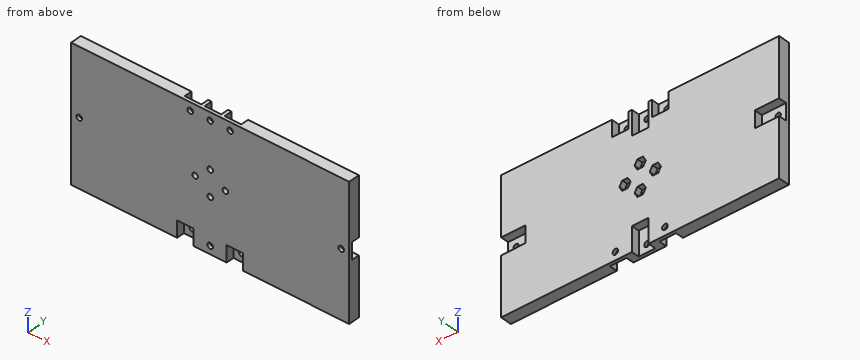
from build123d import *

# Parameters (mm, degrees)
SKETCH1_W           = 174.17
SKETCH1_H           = 83
BOSS_EXTRUDE1_DEPTH = 7
SKETCH2_R           = 1.75
CUT_EXTRUDE1_DEPTH  = 8
SKETCH3_R           = 1.75
CUT_EXTRUDE2_DEPTH  = 8
SKETCH4_W           = 15.4
SKETCH4_H           = 10.4
SKETCH4_W_2         = 10.4
SKETCH4_H_2         = 15.4
CUT_EXTRUDE3_DEPTH  = 5
SKETCH5_W           = 10.4
SKETCH5_H           = 10.4
CUT_EXTRUDE4_DEPTH  = 5
SKETCH6_R           = 1.75
CUT_EXTRUDE5_DEPTH  = 3
CUT_EXTRUDE6_DEPTH  = 3.64
SKETCH9_W           = 10.4
SKETCH9_H           = 10.4
CUT_EXTRUDE7_DEPTH  = 5
SKETCH10_R          = 1.75
CUT_EXTRUDE8_DEPTH  = 3


with BuildPart() as part:
    # Sketch1 → Boss-Extrude1 (new body)
    with BuildSketch(Plane(origin=(0, 0, 0), x_dir=(1, 0, 0), z_dir=(0, 1, 0))):
        with Locations((87.085, 41.5)):
            Rectangle(SKETCH1_W, SKETCH1_H)
    extrude(amount=BOSS_EXTRUDE1_DEPTH)

    # Sketch2 → Cut-Extrude1 (cut, through all)
    with BuildSketch(Plane(origin=(0, 7, 0), x_dir=(1, 0, 0), z_dir=(0, 1, 0))):
        with Locations((87.085, 49.5)):
            Circle(SKETCH2_R)
        with Locations((77.585, 41.5)):
            Circle(SKETCH2_R)
        with Locations((96.585, 41.5)):
            Circle(SKETCH2_R)
        with Locations((87.085, 33.5)):
            Circle(SKETCH2_R)
    extrude(amount=-CUT_EXTRUDE1_DEPTH, mode=Mode.SUBTRACT)

    # Sketch3 → Cut-Extrude2 (cut, through all)
    with BuildSketch(Plane(origin=(0, 7, 0), x_dir=(1, 0, 0), z_dir=(0, 1, 0))):
        with Locations((87.085, 78)):
            Circle(SKETCH3_R)
        with Locations((5, 41.5)):
            Circle(SKETCH3_R)
        with Locations((87.085, 5)):
            Circle(SKETCH3_R)
        with Locations((169.17, 41.5)):
            Circle(SKETCH3_R)
    extrude(amount=-CUT_EXTRUDE2_DEPTH, mode=Mode.SUBTRACT)

    # Sketch4 → Cut-Extrude3 (cut)
    with BuildSketch(Plane(origin=(0, 7, 0), x_dir=(1, 0, 0), z_dir=(0, 1, 0))):
        with Locations((7.5, 41.5)):
            Rectangle(SKETCH4_W, SKETCH4_H)
        with Locations((87.085, 7.5)):
            Rectangle(SKETCH4_W_2, SKETCH4_H_2)
        with Locations((87.085, 75.5)):
            Rectangle(SKETCH4_W_2, SKETCH4_H_2)
        with Locations((166.67, 41.5)):
            Rectangle(SKETCH4_W, SKETCH4_H)
    extrude(amount=-CUT_EXTRUDE3_DEPTH, mode=Mode.SUBTRACT)

    # Sketch5 → Cut-Extrude4 (cut)
    with BuildSketch(Plane(origin=(0, 7, 0), x_dir=(1, 0, 0), z_dir=(0, 1, 0))):
        with Locations((74.585, 5)):
            Rectangle(SKETCH5_W, SKETCH5_H)
        with Locations((99.585, 5)):
            Rectangle(SKETCH5_W, SKETCH5_H)
    extrude(amount=-CUT_EXTRUDE4_DEPTH, mode=Mode.SUBTRACT)

    # Sketch6 → Cut-Extrude5 (cut, through all)
    with BuildSketch(Plane(origin=(0, 2, 0), x_dir=(1, 0, 0), z_dir=(0, 1, 0))):
        with Locations((74.585, 5)):
            Circle(SKETCH6_R)
        with Locations((99.585, 5)):
            Circle(SKETCH6_R)
    extrude(amount=-CUT_EXTRUDE5_DEPTH, mode=Mode.SUBTRACT)

    # Sketch7 → Cut-Extrude6 (cut)
    with BuildSketch(Plane(origin=(0, 7, 0), x_dir=(1, 0, 0), z_dir=(0, 1, 0))):
        Polygon((75.824081679, 44.55), (79.345918321, 44.55), (81.106836642, 41.5), (79.345918321, 38.45), (75.824081679, 38.45), (74.063163358, 41.5), align=None)
        Polygon((85.324081679, 52.55), (88.845918321, 52.55), (90.606836642, 49.5), (88.845918321, 46.45), (85.324081679, 46.45), (83.563163358, 49.5), align=None)
        Polygon((100.106836642, 41.5), (98.345918321, 44.55), (94.824081679, 44.55), (93.063163358, 41.5), (94.824081679, 38.45), (98.345918321, 38.45), align=None)
        Polygon((83.563163358, 33.5), (85.324081679, 30.45), (88.845918321, 30.45), (90.606836642, 33.5), (88.845918321, 36.55), (85.324081679, 36.55), align=None)
    extrude(amount=-CUT_EXTRUDE6_DEPTH, mode=Mode.SUBTRACT)

    # Sketch9 → Cut-Extrude7 (cut)
    with BuildSketch(Plane.XZ):
        with Locations((71.585, -78)):
            Rectangle(SKETCH9_W, SKETCH9_H)
        with Locations((102.585, -78)):
            Rectangle(SKETCH9_W, SKETCH9_H)
    extrude(amount=-CUT_EXTRUDE7_DEPTH, mode=Mode.SUBTRACT)

    # Sketch10 → Cut-Extrude8 (cut, through all)
    with BuildSketch(Plane.XZ.offset(-5)):
        with Locations((71.585, -78)):
            Circle(SKETCH10_R)
        with Locations((102.585, -78)):
            Circle(SKETCH10_R)
    extrude(amount=-CUT_EXTRUDE8_DEPTH, mode=Mode.SUBTRACT)


solid = part.part
Can you work these out from the model? Positions are in its coordinate system, mm. Give positions to 0.01 mm unless a question says otherwise; leave off trailing zeros. Loops run counter-clockwise (first coordinate to the right, second up) from the corner with the lowest first, then second, coordinate; pieces in that order, holes last. Notation, with made-up numbers: (-4, -22.75) - (38, -22.75) arc R30 ccw to (38, 1.25) - close; hole circle Ø10 at (77.5, -16). An arc over 180 degrees is marked (long way). Answer as a JSON object with one key per item and string values.
Q1. Imagine slicing it at A-A on x = 5. Write out the boundary of the cut face in (y, z).
Geometry says:
{"outline": "(0, -83) - (7, -83) - (7, -46.7) - (2, -46.7) - (2, -43.25) - (0, -43.25) - close; (0, -39.75) - (2, -39.75) - (2, -36.3) - (7, -36.3) - (7, 0) - (0, 0) - close"}
Q2. Imagine slicing it at B-B on z = -5. Write out the boundary of the cut face in (x, y) (3 decimals).
Geometry says:
{"outline": "(0, 0) - (72.835, 0) - (72.835, 2) - (69.385, 2) - (69.385, 7) - (0, 7) - close; (76.335, 0) - (85.335, 0) - (85.335, 2) - (81.885, 2) - (81.885, 7) - (79.785, 7) - (79.785, 2) - (76.335, 2) - close; (88.835, 0) - (97.835, 0) - (97.835, 2) - (94.385, 2) - (94.385, 7) - (92.285, 7) - (92.285, 2) - (88.835, 2) - close; (101.335, 0) - (174.17, 0) - (174.17, 7) - (104.785, 7) - (104.785, 2) - (101.335, 2) - close"}
Q3. If I drill on L1, parallel to X at y = 0.55, z = -5 (3 decimals); L2, parallel to X at y = 6.75, z = -70 (3 decimals); L3, parallel to X at y = 1.6, z = -33.5 (3 decimals), over which ranges is the centre line in solid material (lowest first)?
Geometry says:
{"L1": "0 to 72.835, 76.335 to 85.335, 88.835 to 97.835, 101.335 to 174.17", "L2": "0 to 81.885, 92.285 to 174.17", "L3": "0 to 85.335, 88.835 to 174.17"}
Q4. Will these pins go through, and if not, where does the flat tip stop? P1, Ø1.5, axis at x = 69.5, y = 1.5, coming from the -Z side; P2, Ø4, axis at x = 87.5, y = 5.5, coming from the +Z side; P3, Ø4, axis at x = 87.5, y = 6, coming from the -Z side.
Geometry says:
{"P1": "z = -72.8", "P2": "z = -15.2", "P3": "z = -67.8"}
